CAD build for the part. Positions are in the model's coordinates, mm. A direction names the side the tool comes from. Coordinates: 2 decimals unless noted, no trailing zeros. Loops run counter-clockwise (first coordinate to the right, second up) from the corner with the lowest first, then second, coordinate; pieces in that order, holes last. Notation, with made-up numbers: (86.5, -28.5) -> (145.5, -28.5) arc R25 ccw to (145.5, -2.5) -> close; hole circle Ø5 at (8, 32). An arc over 180 degrees is marked (long way). Write item = value, one per line. Start each with the question number.
(1) Pull direction X, two halves, no side cores. Call faces 5 (the face through (16, 0.76, 10.57)), 6 (the face through (10.5, 17.7, -2.8)), 7 (the face through (0, 1, 12)), 8 (the face through (-10.59, 17.54, -0.04)): +X half, -X half, draft (parallel to the pull), parting line (faces both ways), or undercut.
(2) Band-saw the part on A-A (z = -19). Write the cut outline in (x, y), and give its area (3 significant figures).
(3) Tool access for faces 1 (the face through (10.142, 9, -3)), 2 (the face through (-10.4, 17.8, 2.8)), 3 (the face through (-10.6, 7.9, 2.8)), 4 (the face through (-10, 1, -13)): list every direction of +Z, -Z, +X, -X, +Y, -Y with a clear straight run to the whole face (end or side of a thin tool).
(4) Drill centre lines: line 1 (Z direction, x = 2.5, y = 3.5); line 2 (X direction, y = 7, z = -4.5) (1 decimal); line 3 (X direction, y = 4.5, z = -1) (3 decimals). Where is each one in solid material? Low to high. Write a range as from..to.
(5) Band-saw the part on C-C (x = 4.5). Write the cut outline in (y, z), and give its area (3 significant figures).
(6) Flat gauge pins, fed straight in: P1, Ø4, axis at y = 10, z = -3, coming from the +X side (3 decimals); P2, Ø4, axis at y = 14.5, z = -8, coming from the +X side; P3, Ø1, axis at x = 10.5, y = 11.5, coming from the +Z side. Where does each tip first touch, or does it go through?
Autodesk Inventor part; units mm, degrees
ref_plane "YZ Plane" through (0, 0, 0) normal (1, 0, 0) x (0, 1, 0)
ref_plane "XZ Plane" through (0, 0, 0) normal (0, 1, 0) x (-1, 0, 0)
ref_plane "XY Plane" through (0, 0, 0) normal (0, 0, 1) x (1, 0, 0)
sketch "Sketch1" plane through (0, 0, 0) normal (0, 1, 0) x (-1, 0, 0)
  line L0 (-10.1425, -6.7516) -> (10.1425, -6.7516)
  line L1 (10.1425, -6.7516) -> (10.1425, 6.7516)
  line L2 (10.1425, 6.7516) -> (-10.1425, 6.7516)
  line L3 (-10.1425, 6.7516) -> (-10.1425, -6.7516)
  line L4 (-10.1425, -6.7516) -> (10.1425, 6.7516) construction
  line L5 (10.1425, -6.7516) -> (-10.1425, 6.7516) construction
  line L6 (-13.125, -9.7516) -> (13.125, -9.7516)
  line L7 (13.125, -9.7516) -> (13.125, 9.7516)
  line L8 (13.125, 9.7516) -> (-13.125, 9.7516)
  line L9 (-13.125, 9.7516) -> (-13.125, -9.7516)
  point P0 (0, 0)
  point P1 (0, 0)
  point P2 (0, 0)
  point P3 (0, -9.7516)
  point P4 (0, 0)
  point P5 (-13.125, 0)
  point P6 (0, 0)
  dimension "d2" = 19.685
  dimension "d3" = 12.9032
  dimension "d4" = 3
  dimension "d12" = 26.25
extrude "Extrusion1" add sketch "Sketch1" along normal blind 18
sketch "Sketch2" plane through (0, 0, 0) normal (0, -1, 0) x (1, 0, 0)
  line L0 (10.1425, 6.7516) -> (10.1425, -6.7516)
  line L1 (10.1425, -6.7516) -> (-10.1425, -6.7516)
  line L2 (-10.1425, -6.7516) -> (-10.1425, 6.7516)
  line L3 (-10.1425, 6.7516) -> (10.1425, 6.7516)
  line L4 (17.5, -22.7) -> (17.5, 12)
  line L5 (17.5, 12) -> (-17.5, 12)
  line L6 (-17.5, 12) -> (-17.5, -22.7)
  line L7 (13.125, -9.7516) -> (-13.125, -9.7516)
  line L8 (-13.125, 9.7516) -> (13.125, 9.7516)
  line L9 (-13.125, -9.7516) -> (-13.125, 9.7516)
  line L10 (-12, -22.7) -> (-12, -17)
  line L11 (-7, -12) -> (7, -12)
  line L12 (12, -17) -> (12, -22.7)
  line L13 (0, -23.1968) -> (0, 12) construction
  line L14 (-17.5, -22.7) -> (-12, -22.7)
  line L15 (12, -22.7) -> (17.5, -22.7)
  arc A0 (-7, -12) -> (-12, -17) centre (-7, -17) ccw
  arc A1 (12, -17) -> (7, -12) centre (7, -17) ccw
  point P0 (0, 0)
  point P1 (0, 0)
  point P2 (-12, -12)
  point P3 (12, -12)
  dimension "d8" = 35
  dimension "d13" = 12
  dimension "d15" = 2.2484
  dimension "d16" = 2.2484
  dimension "d17" = 22.7
  dimension "d18" = 24
  dimension "d32" = 34.7
  dimension "d33" = 5
extrude "Extrusion2" add sketch "Sketch2" against normal blind 1.5
sketch "Sketch3" plane through (0, 0, 0) normal (0, 0, 1) x (1, 0, 0)
  line L0 (-13.125, 1.5) -> (-13.125, 18)
  line L1 (13.125, 18) -> (-13.125, 18)
  line L2 (-10.1425, 0) -> (-10.1425, 18)
  line L3 (10.1425, 0) -> (10.1425, 18)
  line L4 (13.125, 1.5) -> (13.125, 18)
  line L5 (7, 0) -> (-7, 0)
  line L6 (-11.05, 0) -> (-11.05, 14.5925)
  line L7 (-11.05, 14.5925) -> (-10.1425, 15.5)
  line L8 (11.05, 0) -> (11.05, 14.5925)
  line L9 (11.05, 14.5925) -> (10.1425, 15.5)
  line L10 (0, 18) -> (0, 0) construction
  line L11 (-10.1425, 17.0925) -> (-11.05, 18)
  line L12 (-11.05, 14.5925) -> (-11.05, 18) construction
  line L13 (10.1425, 17.0925) -> (11.05, 18)
  line L14 (11.05, 18) -> (11.05, 14.5925) construction
  line L15 (-10.1425, 0) -> (-11.05, 0)
  line L16 (10.1425, 0) -> (11.05, 0)
  line L17 (-10.1425, 15.5) -> (-10.1425, 0)
  line L18 (10.1425, 0) -> (10.1425, 15.5)
  line L19 (10.1425, 17.0925) -> (10.1425, 18)
  line L20 (10.1425, 18) -> (11.05, 18)
  line L21 (-11.05, 18) -> (-10.1425, 18)
  line L22 (-10.1425, 18) -> (-10.1425, 17.0925)
  dimension "d21" = 2.5
  dimension "d22" = 21.5
  dimension "d24" = 45
  dimension "d34" = 20.285
extrude "Extrusion3" cut sketch "Sketch3" along normal mid plane 5.6
fillet "Fillet1" radius 5 2 edges at (17.5, 0.75, 12) (-17.5, 0.75, 12)
fillet "Fillet2" radius 5 4 edges at (13.125, 9.75, 9.7516) (13.125, 9.75, -9.7516) (-13.125, 9.75, 9.7516) (-13.125, 9.75, -9.7516)
equation "\"d15\" = d16"
properties part number "Switch Holder"
Findings below:
q1.face_5 = +X half
q1.face_6 = undercut
q1.face_7 = draft
q1.face_8 = undercut
q2.outline = (-17.5, 0) -> (-12, 0) -> (-12, 1.5) -> (-17.5, 1.5) -> close; (12, 0) -> (17.5, 0) -> (17.5, 1.5) -> (12, 1.5) -> close
q2.area = 16.5 mm²
q3.face_1 = +Y, -Y
q3.face_2 = +Y
q3.face_3 = -Y
q3.face_4 = -Z, +Y, -Y
q4.line_1 = -9.75..-6.75, 6.75..9.75
q4.line_2 = -13.1..-10.1, 10.1..13.1
q4.line_3 = -13.125..-11.05, 11.05..13.125
q5.outline = (0, -12) -> (1.5, -12) -> (1.5, -9.75) -> (18, -9.75) -> (18, -6.75) -> (0, -6.75) -> close; (0, 6.75) -> (18, 6.75) -> (18, 9.75) -> (1.5, 9.75) -> (1.5, 12) -> (0, 12) -> close
q5.area = 115 mm²
q6.P1 = 13.125
q6.P2 = 12.97
q6.P3 = 9.39
